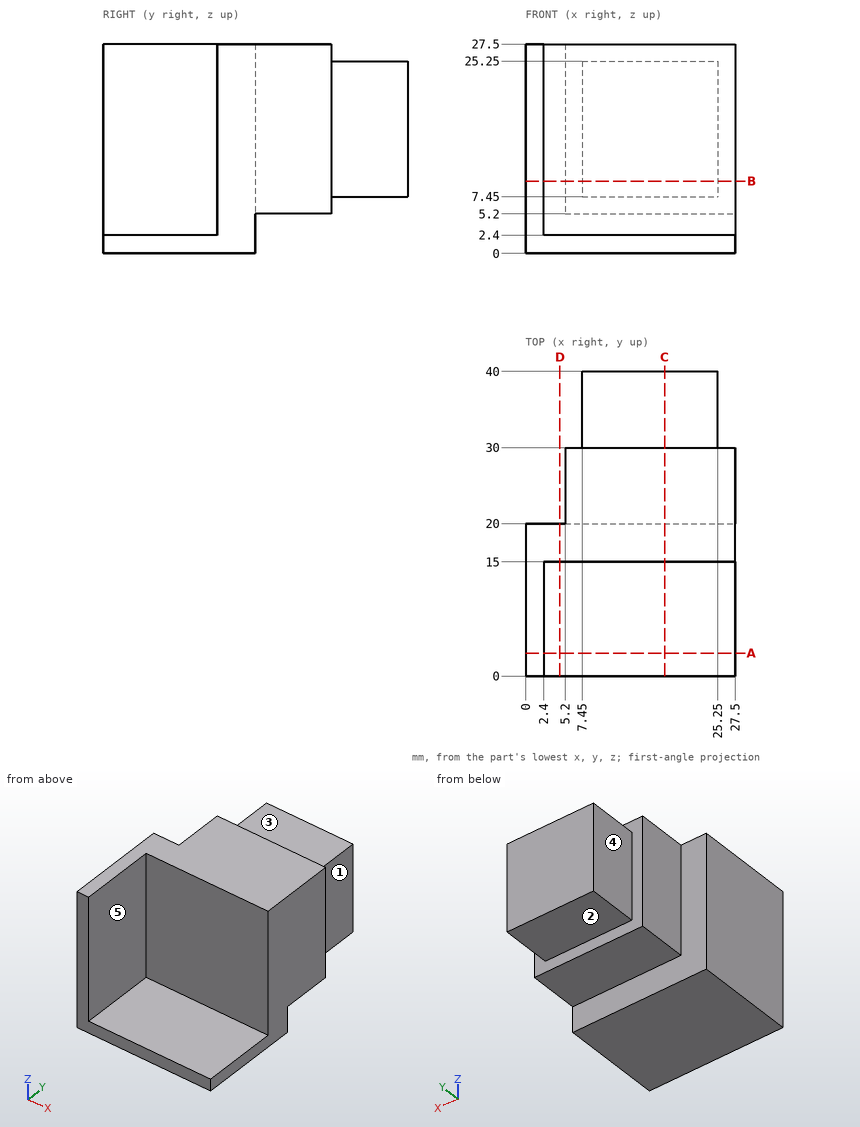
Here's the drawing with two shaded views (mm, measured from the low corner). I have some questions. A direction names the side the tool comes from. Round coordinates to 2 decimals unless told otherwise and drop trailing zeros. Write each loop counter-clockwise with the first axis right and the second up, starting at its lowest first coordinate (ties: lowest second). Pieces come first, ordered by that corner, then holes.
(1) Suppose I cut it at A-A on y = 3. Write out the boundary of the cut face in (x, z), and give its area (3 significant figures).
Findings below:
outline: (0, 0) - (27.5, 0) - (27.5, 2.4) - (2.4, 2.4) - (2.4, 27.5) - (0, 27.5) - close
area: 126 mm2
(2) Suppose I cut it at D-D on x = 4.5. Write out the boundary of the cut face in (y, z), and give its area (4 significant figures).
Findings below:
outline: (0, 0) - (20, 0) - (20, 27.5) - (15, 27.5) - (15, 2.4) - (0, 2.4) - close
area: 173.5 mm2
(3) Suppose I cut it at B-B on z = 9.5. Write out the boundary of the cut face in (x, y), and give its area (4 significant figures).
Findings below:
outline: (0, 0) - (2.4, 0) - (2.4, 15) - (27.5, 15) - (27.5, 30) - (25.25, 30) - (25.25, 40) - (7.45, 40) - (7.45, 30) - (5.2, 30) - (5.2, 20) - (0, 20) - close
area: 574.5 mm2
(4) If I drill on probe 1 along X at (y, z) = (3.5, 9.25); probe 2 along X at (y, z) = (28.5, 13.75); probe 3 along Y at (x, z) = (19.5, 14.5), over which ranges is the centre line in solid material (lowest first)?
Findings below:
probe 1: x = 0 to 2.4
probe 2: x = 5.2 to 27.5
probe 3: y = 15 to 40
(5) Suppose I cut it at C-C on x = 18.25. Write out the boundary of the cut face in (y, z).
Findings below:
outline: (0, 0) - (20, 0) - (20, 5.2) - (30, 5.2) - (30, 7.45) - (40, 7.45) - (40, 25.25) - (30, 25.25) - (30, 27.5) - (15, 27.5) - (15, 2.4) - (0, 2.4) - close
(6) Which directions (+Z, -Z, +X, -X, +Y, -Y) give clear straight access to the entire face, cutting with the end or side of a thin tool? Please do the marked faces 1, 2, 3, 4 and 5.
Findings below:
face 1: +Z, -Z, +X, +Y
face 2: -Z, +X, -X, +Y
face 3: +Z, +X, -X, +Y
face 4: +Z, -Z, -X, +Y
face 5: +Z, +X, -Y
(7) For pin 1 (8 mm diameter, centred on y = 37, z = 20, fed in from -X); pin 2 (4.5 mm diameter, centred on y = 8, z = 15.5, fed in from +X); pin 3 (1.5 mm diameter, centred on x = 10.5, y = 28.5, fed in from -Z); pin 4 (1 mm diameter, centred on y = 31, z = 6, fed in from +X), each with a flat end and sliding along its axis, tell me the tip position at first contact or that it passes through.
Findings below:
pin 1: stops at x = 7.45
pin 2: stops at x = 2.4
pin 3: stops at z = 5.2
pin 4: passes through
